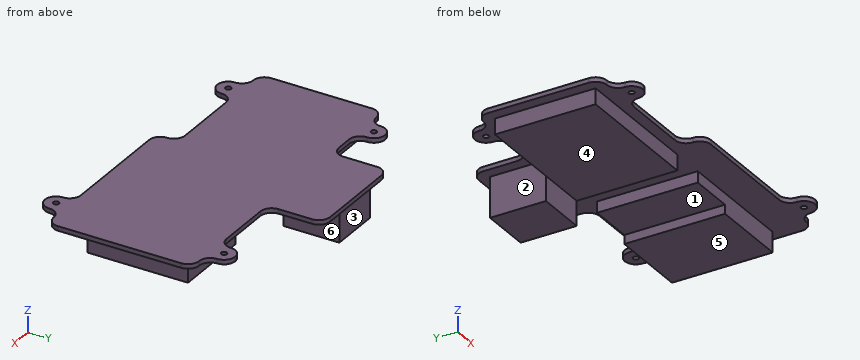
```python
from build123d import *

# Parameters (mm, degrees)
F2_DEPTH = 2
F3_DEPTH = 9
F4_DEPTH = 5
F0_W     = 22.5
F0_H     = 25
F5_DEPTH = 18
F6_DEPTH = 7
F7_D     = 2.5


with BuildPart() as f2:
    # F1 (on Top) → F2 (new body)
    with BuildSketch(Plane.XY):
        with BuildLine():
            ThreePointArc((70, -5), (73.5355339059, -3.5355339059), (75, 0))
            Line((75, 0), (75, 55))
            ThreePointArc((75, 55), (73.5355339059, 58.5355339059), (70, 60))
            ThreePointArc((70, 60), (66.4644660941, 61.4644660941), (65, 65))
            ThreePointArc((65, 65), (63.5355339059, 68.5355339059), (60, 70))
            ThreePointArc((60, 70), (56.4644660941, 68.5355339059), (55, 65))
            ThreePointArc((55, 65), (53.5355339059, 61.4644660941), (50, 60))
            Line((50, 60), (25, 60))
            ThreePointArc((25, 60), (21.4644660941, 61.4644660941), (20, 65))
            Line((20, 65), (20, 80))
            ThreePointArc((20, 80), (18.5355339059, 83.5355339059), (15, 85))
            Line((15, 85), (-22.5, 85))
            ThreePointArc((-22.5, 85), (-26.0355339059, 83.5355339059), (-27.5, 80))
            Line((-27.5, 80), (-27.5, 65))
            ThreePointArc((-27.5, 65), (-28.9644660941, 61.4644660941), (-32.5, 60))
            Line((-32.5, 60), (-40, 60))
            ThreePointArc((-40, 60), (-43.5355339059, 61.4644660941), (-45, 65))
            ThreePointArc((-45, 65), (-46.4644660941, 68.5355339059), (-50, 70))
            ThreePointArc((-50, 70), (-53.5355339059, 68.5355339059), (-55, 65))
            ThreePointArc((-55, 65), (-56.4644660941, 61.4644660941), (-60, 60))
            ThreePointArc((-60, 60), (-63.5355339059, 58.5355339059), (-65, 55))
            Line((-65, 55), (-65, 10))
            ThreePointArc((-65, 10), (-63.5355339059, 6.4644660941), (-60, 5))
            ThreePointArc((-60, 5), (-56.4644660941, 3.5355339059), (-55, 0))
            ThreePointArc((-55, 0), (-53.5355339059, -3.5355339059), (-50, -5))
            ThreePointArc((-50, -5), (-46.4644660941, -3.5355339059), (-45, 0))
            ThreePointArc((-45, 0), (-43.5355339059, 3.5355339059), (-40, 5))
            Line((-40, 5), (-10, 5))
            ThreePointArc((-10, 5), (-6.4644660941, 3.5355339059), (-5, 0))
            ThreePointArc((-5, 0), (-3.5355339059, -3.5355339059), (0, -5))
            Line((0, -5), (50, -5))
            ThreePointArc((50, -5), (53.5355339059, -6.4644660941), (55, -10))
            ThreePointArc((55, -10), (56.4644660941, -13.5355339059), (60, -15))
            ThreePointArc((60, -15), (63.5355339059, -13.5355339059), (65, -10))
            ThreePointArc((65, -10), (66.4644660941, -6.4644660941), (70, -5))
        make_face()
        Polygon((-22.5, 55), (-22.5, 80), (15, 80), (15, 55), (70, 55), (70, 0), (0, 0), (0, 10), (-60, 10), (-60, 55), align=None, mode=Mode.SUBTRACT)
        Polygon((15, 80), (-22.5, 80), (-22.5, 55), (-60, 55), (-60, 10), (0, 10), (0, 0), (70, 0), (70, 55), (15, 55), align=None)
    extrude(amount=F2_DEPTH)

    # F0 (on Top) → F3 (join)
    with BuildSketch(Plane.XY):
        Polygon((35, 55), (35, 10), (70, 10), (70, 55), (40, 55), align=None)
    extrude(amount=-F3_DEPTH)

    # F0 (on Top) → F4 (join)
    with BuildSketch(Plane.XY):
        Polygon((15, 40), (15, 10), (35, 10), (35, 55), (15, 55), align=None)
    extrude(amount=-F4_DEPTH)

    # F0 (on Top) → F5 (join)
    with BuildSketch(Plane.XY):
        with Locations((-11.25, 67.5)):
            Rectangle(F0_W, F0_H)
    extrude(amount=-F5_DEPTH)

    # F0 (on Top) → F6 (join)
    with BuildSketch(Plane.XY):
        Polygon((-60, 10), (0, 10), (0, 40), (0, 55), (-22.5, 55), (-60, 55), align=None)
    extrude(amount=-F6_DEPTH)

    # F7 (through all)
    with Locations(Plane(origin=(0, 0, 0), x_dir=(1, 0, 0), z_dir=(0, 0, -1))):
        with Locations((60, -65), (-50, -65), (-50, 0), (60, 10)):
            Hole(F7_D / 2)


solid = f2.part
```
Work out the finished part from the listing and answer in its coordinate system (mm). Face numbers are marked on the shaded views. A direction names the side the tool comes from. Coordinates: 2 decimals unless noted, no trailing zeros. Loops run counter-clockwise (first coordinate to the right, second up) from the corner with the lowest first, then second, coordinate; pieces in that order, holes last. Notation, with made-up numbers: (11.25, 8.25) - (66.25, 8.25) arc R27 ccw to (66.25, 35.25) - close; hole circle Ø7 at (-29.5, 48.5). An arc over 180 degrees is marked (long way). Use a Markdown table: item, result.
Item 1: Find section B-B, the plane y = 38.5. Determine the outline of the cut face in (x, z).
Evaluation:
| item | result |
|---|---|
| outline | (-65, 0) - (-60, 0) - (-60, -7) - (0, -7) - (0, 0) - (15, 0) - (15, -5) - (35, -5) - (35, -9) - (70, -9) - (70, 0) - (75, 0) - (75, 2) - (-65, 2) - close |
Item 2: Find section C-C, the plane y = 68.5. Determine the outline of the cut face in (x, z).
Evaluation:
| item | result |
|---|---|
| outline | (-53.57, 0) - (-46.43, 0) - (-46.43, 2) - (-53.57, 2) - close; (-27.5, 0) - (-22.5, 0) - (-22.5, -18) - (0, -18) - (0, 0) - (20, 0) - (20, 2) - (-27.5, 2) - close; (56.43, 0) - (63.57, 0) - (63.57, 2) - (56.43, 2) - close |
Item 3: For the marked faces 4, 5 and 6, determine the directions among +Z, -Z, +X, -X, +Y, -Y from which every point of the face is accessible in a straight line to the end or side of a thin tool.
Evaluation:
| item | result |
|---|---|
| face 4 | -Z, -X, -Y |
| face 5 | -Z, +X, -X, +Y, -Y |
| face 6 | -Z, +Y, -Y |
Item 4: Find section D-D, the plane x = 48.5. Determine the outline of the cut face in (y, z).
Evaluation:
| item | result |
|---|---|
| outline | (-5, 0) - (10, 0) - (10, -9) - (55, -9) - (55, 0) - (60, 0) - (60, 2) - (-5, 2) - close |
Item 5: Given pin 1 Ø6 at (y, z) = (28.5, -10) entering from +X; pin 2 Ø1.5 at (x, y) = (-50, 0) entering from +Z; pin 3 Ø9 at (y, z) = (69, -13.5) entering from -X; pin 4 Ø2 at (y, z) = (39, -5) entering from -X, each flat-ended and moving along its own axis, determine where each tip first touches the part or whether it passes through.
Evaluation:
| item | result |
|---|---|
| pin 1 | stops at x = 70 |
| pin 2 | passes through |
| pin 3 | stops at x = -22.5 |
| pin 4 | stops at x = -60 |
Item 6: Consider probe 1 along Y at (x, z) = (-50, 1.5); probe 2 along Y at (x, z) = (60, 0.5); probe 3 along X at (y, z) = (65, 0.65). Determine where each line is inside the solid, lowest interval first. Write a range as from..to.
Evaluation:
| item | result |
|---|---|
| probe 1 | y = -5..-1.25, 1.25..63.75, 66.25..70 |
| probe 2 | y = -15..-11.25, -8.75..63.75, 66.25..70 |
| probe 3 | x = -55..-51.25, -48.75..-45, -27.5..20, 55..58.75, 61.25..65 |
Item 7: The mould has two halves that part along X. Classify the marked faces 1, 2 and 3: +X half, -X half, draft (parallel to the pull), parting line (faces both ways), or undercut.
Evaluation:
| item | result |
|---|---|
| face 1 | undercut |
| face 2 | -X half |
| face 3 | draft |
Item 8: Find section A-A, the plane z = -2.5. Determine the outline of the cut face in (x, y), and give its area (3 significant figures).
Evaluation:
| item | result |
|---|---|
| outline | (-60, 10) - (0, 10) - (0, 80) - (-22.5, 80) - (-22.5, 55) - (-60, 55) - close; (15, 10) - (70, 10) - (70, 55) - (15, 55) - close |
| area | 5,740 mm2 |
